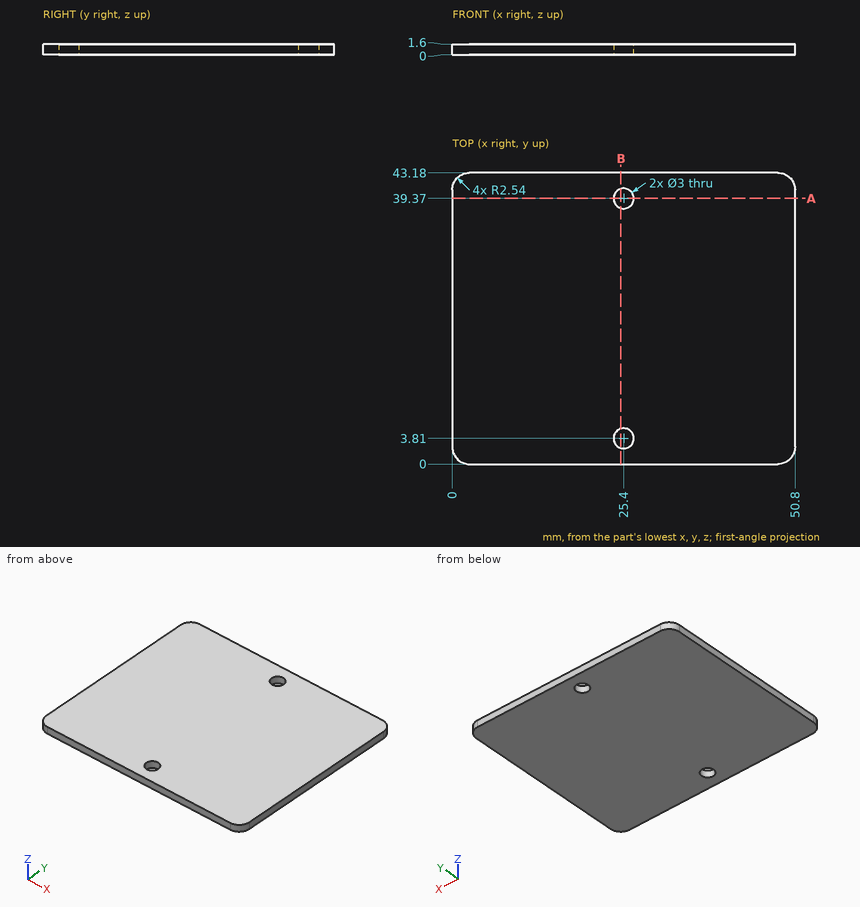
Geometry check sheet. Reference: drawing and pictorial views, mm from the part's lowest x, y, z. Coordinates: 2 decimals unless noted, no trailing zeros. Write each loop counter-clockwise with the first axis right and the second up, starting at its lowest first coordinate (ties: lowest second). Pieces come first, ordered by that corner, then holes. Notation, with made-up numbers: (31.5, 1) - (67.5, 1) arc R7 cw to (67.5, 10) - close; hole circle Ø5 at (-17.5, 34). An arc over 180 degrees is marked (long way). One line per question, with ' | ' between items. Start each with the question number.
1. Gauge pin test, flat end, axial feed: P1, Ø4, axis at x = 25.4, y = 3.81, coming from the +Z side. Record the tip position at first contact, or that the pin passes through.
2. Section check B-B (x = 25). Enter the section's corners in (y, z), plus the area to 3 significant figures.
3. Section check A-A (y = 39.37). Enter the section's corners in (x, z).
4. Material ranges on line 1 along Y through (x, z) = (25.5, 1.55); line 2 along Y through (x, z) = (26.5, 0.8); line 3 along X through (y, z) = (39.5, 1.45), recorded low to high.
Computed values:
1) P1: z = 1.6
2) outline: (0, 0) - (2.36, 0) - (2.36, 1.6) - (0, 1.6) - close; (5.26, 0) - (37.92, 0) - (37.92, 1.6) - (5.26, 1.6) - close; (40.82, 0) - (43.18, 0) - (43.18, 1.6) - (40.82, 1.6) - close | area: 59.8 mm²
3) outline: (0, 0) - (23.9, 0) - (23.9, 1.6) - (0, 1.6) - close; (26.9, 0) - (50.8, 0) - (50.8, 1.6) - (26.9, 1.6) - close
4) line 1: 0 to 2.31, 5.31 to 37.87, 40.87 to 43.18 | line 2: 0 to 2.79, 4.83 to 38.35, 40.39 to 43.18 | line 3: 0 to 23.91, 26.89 to 50.8
